Can you work these out from the drawing? Everything is in mm from the part's minimum corner. Round coordinates to 2 decimals unless told otherwise and drop trailing zeros. Loops run counter-clockwise (first coordinate to the right, second up) from the corner with the lowest first, then second, coordinate; pieces in that order, holes last. Notation, with made-up numbers: M 48.25,71.5 L 107.25,71.5 A21 ccw 107.25,85.5 Z; hole C -25.75,75.5 d5. An arc over 180 degrees is marked long. Answer in a Markdown table with one row per item.
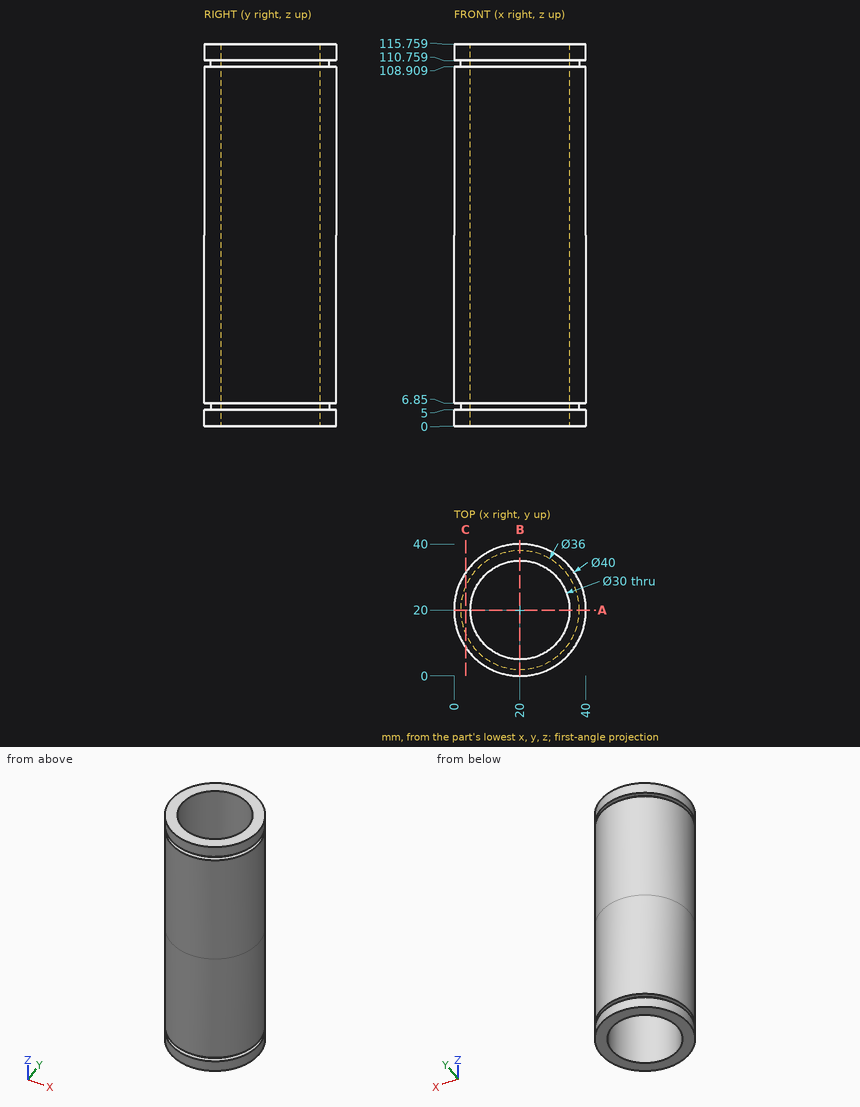
1) I want a section at C-C, the plane x = 3.5. Please give me the cut outline in (y, z), plus the area to 3 significant figures.
Computed:
| item | result |
|---|---|
| outline | M 8.7,0 L 31.3,0 L 31.3,5 L 27.19,5 L 27.19,6.85 L 31.3,6.85 L 31.3,108.91 L 27.19,108.91 L 27.19,110.76 L 31.3,110.76 L 31.3,115.76 L 8.7,115.76 L 8.7,110.76 L 12.81,110.76 L 12.81,108.91 L 8.7,108.91 L 8.7,6.85 L 12.81,6.85 L 12.81,5 L 8.7,5 Z |
| area | 2,590 mm² |
2) I want a section at A-A, the plane y = 20. Please give me the cut outline in (x, z).
Computed:
| item | result |
|---|---|
| outline | M 0,0 L 5,0 L 5,115.76 L 0,115.76 L 0,110.76 L 2,110.76 L 2,108.91 L 0,108.91 L 0,6.85 L 2,6.85 L 2,5 L 0,5 Z; M 35,0 L 40,0 L 40,5 L 38,5 L 38,6.85 L 40,6.85 L 40,108.91 L 38,108.91 L 38,110.76 L 40,110.76 L 40,115.76 L 35,115.76 Z |
3) Will these pins go through, and if not, where does the flat tip stop? P1, Ø5, axis at x = 35.5, z = 46, coming from the -Y side; P2, Ø1, axis at x = 25, z = 29.5, coming from the -Y side; P3, Ø12, axis at x = 8.5, z = 22.5, coming from the +Y side.
Computed:
| item | result |
|---|---|
| P1 | stops at y = 4.8 |
| P2 | stops at y = 0.51 |
| P3 | stops at y = 39.23 |
4) I need wall thicknesses on line 1 (Z direction, x = 2, y = 13.5); line 2 (Y direction, x = 20, z = 57); line 3 (X direction, y = 28, z = 48). Which ranges of each line are inside material? Lowest first, please.
Computed:
| item | result |
|---|---|
| line 1 | z = 0 to 5, 6.85 to 108.91, 110.76 to 115.76 |
| line 2 | y = 0 to 5, 35 to 40 |
| line 3 | x = 1.67 to 7.31, 32.69 to 38.33 |
